Autodesk Inventor part; units mm, degrees
ref_plane "YZ Plane" through (0, 0, 0) normal (1, 0, 0) x (0, 1, 0)
ref_plane "XZ Plane" through (0, 0, 0) normal (0, 1, 0) x (-1, 0, 0)
ref_plane "XY Plane" through (0, 0, 0) normal (0, 0, 1) x (1, 0, 0)
sketch "Skizze1" plane through (0, 0, 0) normal (0, 0, 1) x (1, 0, 0)
  line L0 (0, 0) -> (80, 0)
  line L1 (80, 0) -> (80, 50)
  line L2 (80, 50) -> (0, 50)
  line L3 (0, 50) -> (0, 0)
  dimension "Breite" = 50
  dimension "Laenge" = 80
extrude "Extrusion1" add sketch "Skizze1" along normal blind 7
chamfer "Fasen1" distance 3 angle 45 4 edges at (80, 50, 3.5) (80, 0, 3.5) (0, 50, 3.5) (0, 0, 3.5)
sketch "Skizze2" plane through (0, 0, 7) normal (0, 0, 1) x (1, 0, 0)
  line L0 (77, 50) -> (3, 50)
  line L1 (40, 50) -> (40, 0) construction
  line L2 (0, 47) -> (0, 3)
  line L3 (0, 25) -> (80, 25) construction
  line L4 (80, 3) -> (80, 47)
  point P0 (0, 0)
  point P1 (13, 36)
  dimension "Punktabstand1" = 13
  dimension "Punktabstand2" = 14
hole "Bohrung1" at (13, 36, 7) direction (0, 0, -1) diameter 5.9175 end through all
sketch "Skizze3" plane through (0, 0, 7) normal (0, 0, 1) x (1, 0, 0)
  line L0 (30, 25) -> (50, 25) construction
  line L1 (30, 22) -> (50, 22)
  line L2 (50, 28) -> (30, 28)
  arc A0 (30, 28) -> (30, 22) centre (30, 25) ccw
  arc A1 (50, 22) -> (50, 28) centre (50, 25) ccw
  line L3 (3, 0) -> (77, 0)
  line L4 (0, 47) -> (0, 3)
  point P0 (0, 0)
  point P1 (40, 25)
  point P2 (40, 0)
  point P3 (0, 25)
  point P4 (40, 0)
  point P5 (0, 25)
  dimension "Mannlochbreite" = 6
  dimension "Mannlochlaenge" = 20
extrude "Extrusion2" cut sketch "Skizze3" against normal blind 2.5
pattern_linear "Rechteckige Anordnung2" count 2 spacing 24 along (0, -1, 0) count 2 spacing 24 along (1, 0, 0) of "Bohrung1"
equation "\"d27\" = Abstand_Zeilen"
equation "\"d30\" = Abstand_Zeilen"
equation "\"Abstand_Zeilen\" = Breite - 2 * Punktabstand1"
equation "\"Abstand_Spalten\" = Laenge - 2 * Punktabstand2"
properties part number "variante-03" material "Edelstahl"
Model file for the job. Use its own axes, mm. A direction names the side the tool comes from. Round coordinates to 2 decimals unless told otherwise and drop trailing zeros. Loops run counter-clockwise (first coordinate to the right, second up) from the corner with the lowest first, then second, coordinate; pieces in that order, holes last. Notation, with made-up numbers: M 16.25,78.5 L 58.25,78.5 A6 ccw 58.25,85.5 Z; hole C 7.5,49 d11. An arc over 180 degrees is marked long. Put each result on its own line as item: value. Start each with the question number.
Item 1: Cut at D-D (y = 25). List the corners of the cut face in (x, z).
Item 2: Cut at B-B (x = 13). List the corners of the cut face in (y, z), then the cut area to 3 significant figures.
Item 3: Drop flat-ended pins along their axis: P1, Ø3.5, axis at x = 13, y = 12, coming from the +Z side; P2, Ø1.8, axis at x = 40.5, y = 24, coming from the +Z side. Give the stop position or say it passes through.
Item 4: Cut at C-C (z = 3.5). List the corners of the cut face in (x, y), then the cut area to 3 significant figures.
Item 5: 3-axis set-ups, long thin cutter, end or side, ignore diameter. For faces 4 (the face through (79, 48, 3)), 5 (the face through (40, 25, 4.5)): which of +Z, -Z, +X, -X, +Y, -Y reach the whole face in a straight line?
Item 6: Mould opens along Y. For faces 1 (the face through (39, 20, 7)), 2 (the face through (12.11, 9.18, 3.45)), 3 (the face through (2, 49, 3)) say: released by +Y, released by -Y, zero draft, split by the parting line, or undercut.
Item 7: Cut at A-A (y = 36). List the corners of the cut face in (x, z), then the cut area to 3 significant figures.
Item 8: Drill centre lines: line 1 along X through (y, z) = (36, 5.75); line 2 along Y through (x, z) = (13, 4); line 3 along Z through (x, y) = (33, 24). Where is each one in solid material? Low to high.
Answer block:
1. outline: M 0,0 L 80,0 L 80,7 L 53,7 L 53,4.5 L 27,4.5 L 27,7 L 0,7 Z
2. outline: M 0,0 L 9.04,0 L 9.04,7 L 0,7 Z; M 14.96,0 L 33.04,0 L 33.04,7 L 14.96,7 Z; M 38.96,0 L 50,0 L 50,7 L 38.96,7 Z
2. area: 267 mm2
3. P1: through
3. P2: z = 4.5
4. outline: M 0,3 L 3,0 L 77,0 L 80,3 L 80,47 L 77,50 L 3,50 L 0,47 Z; hole C 13,12 d5.92; hole C 13,36 d5.92; hole C 37,12 d5.92; hole C 37,36 d5.92
4. area: 3,870 mm2
5. face 4: +Z, -Z, +X, +Y
5. face 5: +Z
6. face 1: zero draft
6. face 2: undercut
6. face 3: released by +Y
7. outline: M 0,0 L 10.04,0 L 10.04,7 L 0,7 Z; M 15.96,0 L 34.04,0 L 34.04,7 L 15.96,7 Z; M 39.96,0 L 80,0 L 80,7 L 39.96,7 Z
7. area: 477 mm2
8. line 1: 0 to 10.04, 15.96 to 34.04, 39.96 to 80
8. line 2: 0 to 9.04, 14.96 to 33.04, 38.96 to 50
8. line 3: 0 to 4.5
